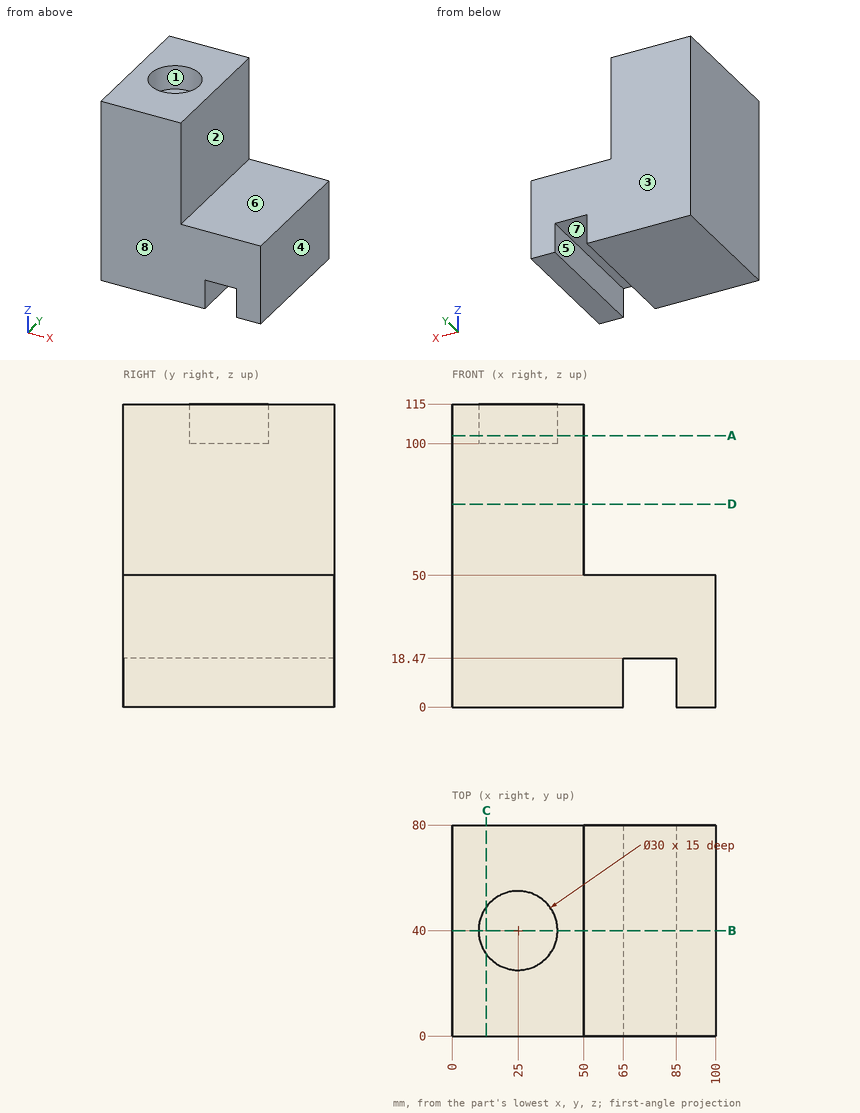
Design review of the part shown in the three views and the two pictorial views. Dimensions are in mm from the part's minimum x, y and z. A direction names the side the tool comes from. Round coordinates to 2 decimals unless told otherwise and drop trailing zeros. Write each loop counter-clockwise with the first axis right and the second up, starting at its lowest first coordinate (ties: lowest second). Pieces come first, ordered by that corner, then holes. Notation, with made-up numbers: (47.25, 89.25) -> (64.25, 89.25) arc R16 cw to (64.25, 120.25) -> close; hole circle Ø4 at (-17.75, -32). An arc over 180 degrees is marked (long way). Answer as a JSON object with one key per item and string values.
1. Clearance check with flat-ended pins moving along their axes: pin 1 (18 mm diameter, centred on x = 25, y = 40, fed in from +Z); pin 2 (1 mm diameter, centred on y = 60, z = 55.5, fed in from +X); pin 3 (10 mm diameter, centred on x = 73.5, y = 57, fed in from -Z); pin 4 (1.5 mm diameter, centred on x = 40.5, y = 70, fed in from -Z). State where each tip first meets the part, or that it passes through.
Results found:
{"pin 1": "stops at z = 100", "pin 2": "stops at x = 50", "pin 3": "stops at z = 18.47", "pin 4": "stops at z = 0"}
2. We need section A-A on z = 103. State the section outline as (x, y) points, and give its area (3 significant figures).
Results found:
{"outline": "(0, 0) -> (50, 0) -> (50, 80) -> (0, 80) -> close; hole circle Ø30 at (25, 40)", "area": "3,290 mm^2"}
3. We need section D-D on z = 77. State the section outline as (x, y) points.
Results found:
{"outline": "(0, 0) -> (50, 0) -> (50, 80) -> (0, 80) -> close"}
4. To check wall thickness, follow line 1 along Y through (x, z) = (25, 105); line 2 along X through (y, z) = (44, 5); line 3 along X through (y, z) = (60.5, 89). State the ranges of each line that lie inside material, in increasing order.
Results found:
{"line 1": "y = 0 to 25, 55 to 80", "line 2": "x = 0 to 65, 85 to 100", "line 3": "x = 0 to 50"}
5. The part is to be moulded in two halves that separate along Z. For the marked faces 6, 7 and 8, say which applies: pulls with the +Z half, pulls with the -Z half, needs draft (parallel to the pull), parting line crosses it, or undercut.
Results found:
{"face 6": "pulls with the +Z half", "face 7": "pulls with the -Z half", "face 8": "needs draft"}
6. We need section B-B on y = 40. State the section outline as (x, z) points, and give its area (3 significant figures).
Results found:
{"outline": "(0, 0) -> (65, 0) -> (65, 18.47) -> (85, 18.47) -> (85, 0) -> (100, 0) -> (100, 50) -> (50, 50) -> (50, 115) -> (40, 115) -> (40, 100) -> (10, 100) -> (10, 115) -> (0, 115) -> close", "area": "7,430 mm^2"}
7. Machinability: for the marked faces 1, 2, 3, 4 and 5, which of the approach directions +Z, -Z, +X, -X, +Y, -Y give a long, thin tool a straight path to every point of the face, cutting with its end or side? Answer none if there is none.
Results found:
{"face 1": "+Z", "face 2": "+Z, +X, +Y, -Y", "face 3": "+Z, -Z, +X, -X, +Y", "face 4": "+Z, -Z, +X, +Y, -Y", "face 5": "-Z, +Y, -Y"}
8. We need section C-C on x = 13. State the section outline as (y, z) points.
Results found:
{"outline": "(0, 0) -> (80, 0) -> (80, 115) -> (49, 115) -> (49, 100) -> (31, 100) -> (31, 115) -> (0, 115) -> close"}
